```python
from build123d import *

# Parameters (mm, degrees)
F0_R     = 4
F1_DEPTH = 1.5
F2_R     = 6
F3_DEPTH = 10
F4_R     = 2.5
F5_DEPTH = 2
F6_R     = 2


with BuildPart() as f1:
    # F0 (on Top) → F1 (new body, symmetric)
    with BuildSketch(Plane.XY):
        with Locations((0.096983, 0.290948)):
            Circle(F0_R)
    extrude(amount=F1_DEPTH, both=True)

    # F2 (on face) → F3 (join)
    with BuildSketch(Plane.XY.offset(1.5)):
        Circle(F2_R)
    extrude(amount=F3_DEPTH)

    # F4 (on face) → F5 (join)
    with BuildSketch(Plane.XY.offset(11.5)):
        Circle(F4_R)
    extrude(amount=F5_DEPTH)

    # F6
    f6_edges = [f1.edges().sort_by_distance(p)[0] for p in [
        (-6, 0, 1.5),
        (-6, 0, 11.5),
    ]]
    fillet(f6_edges, radius=F6_R)


solid = f1.part
```
Here's how the part is built. I have some questions about the finished solid (model axes, mm). A direction names the side the tool comes from. Coordinates: 2 decimals unless noted, no trailing zeros. Write each loop counter-clockwise with the first axis right and the second up, starting at its lowest first coordinate (ties: lowest second). Pieces come first, ordered by that corner, then holes. Notation, with made-up numbers: (1, 68) -> (47, 68) arc R18 cw to (47, 93) -> close; hole circle Ø1 at (86, 40.25). An arc over 180 degrees is marked (long way). Use a Markdown table: item, result. Add a question column.
(1) Please list where these lines run through material, in increasing order: line 1 (Z direction, x = 1.5, y = 3); line 2 (X direction, y = 0.75, z = 10.5); line 3 (Y direction, x = 2.5, z = 4).
(2) For faces 1 (the cylindrical face through (-0.77, -3.614, 0.021)), 2 (the flat face through (0, 0, 13.5)), 3 (the flat face through (2, 2, 11.5)), which set-ups out of +Z, -Z, +X, -X, +Y, -Y let a thin tool reach every point of the face, with its end or its side?
(3) If we section it at A-A, the plane z = 12: Write out the boundary of the cut face in (x, y), and give its area (3 significant figures).
(4) If we section it at B-B, the plane z = 6.5: Write out the boundary of the cut face in (x, y).
(5) I'm going to push flat-ended pins straight in: P1, Ø6, axis at y = 2, z = 12, coming from the -X side; P2, Ø3, axis at x = 2, z = 2.5, coming from the -Y side; P3, Ø3, axis at x = 4.5, z = 12, coming from the -Y side; P4, Ø2, axis at x = 2, y = 2, coming from the +Z side. Where does each tip first touch, or does it pass through?
Outcome:
| question | item | result |
|---|---|---|
| 1 | line 1 | z = -1.5 to 11.5 |
| 1 | line 2 | x = -5.68 to 5.68 |
| 1 | line 3 | y = -5.45 to 5.45 |
| 2 | face 1 | -Z |
| 2 | face 2 | +Z, +X, -X, +Y, -Y |
| 2 | face 3 | +Z |
| 3 | outline | circle Ø5 at (0, 0) |
| 3 | area | 19.6 mm^2 |
| 4 | outline | circle Ø12 at (0, 0) |
| 5 | P1 | stops at x = -5.99 |
| 5 | P2 | stops at y = -5.95 |
| 5 | P3 | stops at y = -4.18 |
| 5 | P4 | stops at z = 13.5 |
